Geometry check sheet. Reference: drawing and pictorial views, mm from the part's lowest x, y, z. Give positions to 0.01 mm unless a question says otherwise; leave off trailing zeros. Write each loop counter-clockwise with the first axis right and the second up, starting at its lowest first coordinate (ties: lowest second). Pieces come first, ordered by that corner, then holes. Notation, with made-up numbers: (81, 43.5) -> (96, 43.5) arc R20 cw to (96, 70.5) -> close; hole circle Ø2 at (31, 46.5). An arc over 180 degrees is marked (long way). Use a Markdown table: item, result. Add a question column.
1. Scan lines: probe 1 along Y at (x, z) = (24.5, 1.85); probe 2 along X at (y, z) = (3.25, 1.35). Record each from-to range of solid material in increasing order. Write a range as [from, to].
2. Gauge pin test, flat ends, axial feed: P1, Ø1, axis at x = 25.5, z = 3.5, coming from the -Y side; P2, Ø0.7, axis at y = 8, z = 3.5, coming from the +X side. Record the tip position at first contact, or that the pin passes through.
3. Cross-section at C-C (y = 3). Enter the section's corners in (x, z).
4. Release check for a two-part mould opening along Y. For the marked faces 1, 2, 3 and 4 record: released by +Y, released by -Y, zero draft, split by the parting line, or undercut.
5. Cross-section at A-A (x = 24.25). Enter the section's corners in (y, z), then the cut area to 3 significant figures.
6. Cross-section at B-B (z = 0.6). Enter the section's corners in (x, y).
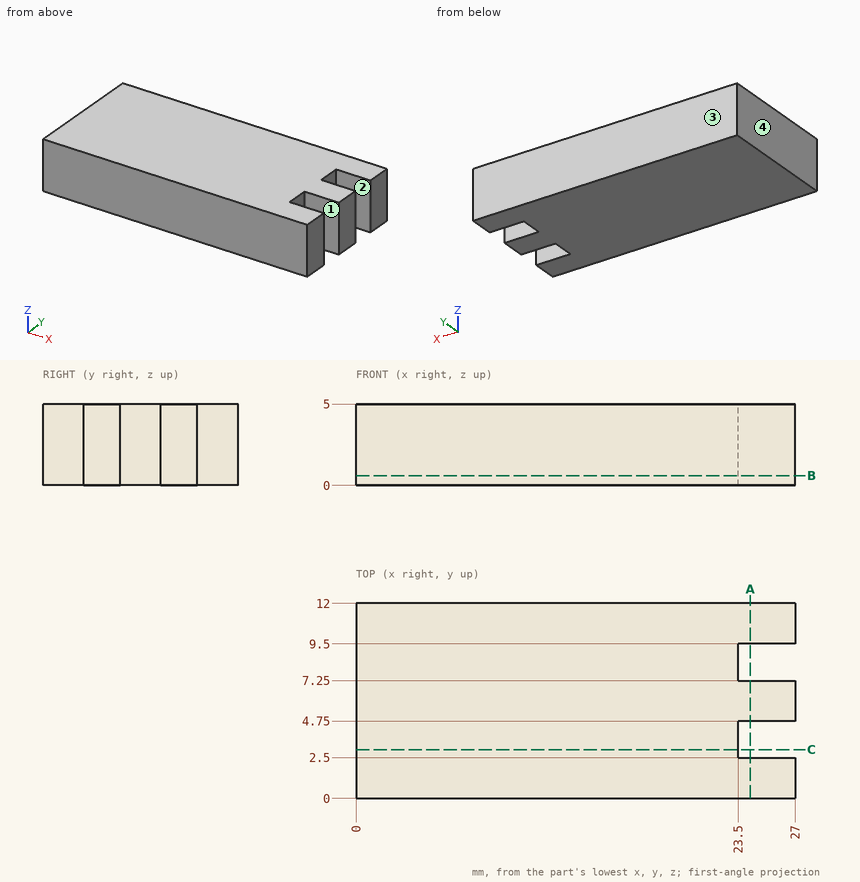
Worked answers:
| question | item | result |
|---|---|---|
| 1 | probe 1 | y = [0, 2.5], [4.75, 7.25], [9.5, 12] |
| 1 | probe 2 | x = [0, 23.5] |
| 2 | P1 | stops at y = 0 |
| 2 | P2 | stops at x = 23.5 |
| 3 | outline | (0, 0) -> (23.5, 0) -> (23.5, 5) -> (0, 5) -> close |
| 4 | face 1 | undercut |
| 4 | face 2 | undercut |
| 4 | face 3 | released by +Y |
| 4 | face 4 | zero draft |
| 5 | outline | (0, 0) -> (2.5, 0) -> (2.5, 5) -> (0, 5) -> close; (4.75, 0) -> (7.25, 0) -> (7.25, 5) -> (4.75, 5) -> close; (9.5, 0) -> (12, 0) -> (12, 5) -> (9.5, 5) -> close |
| 5 | area | 37.5 mm² |
| 6 | outline | (0, 0) -> (27, 0) -> (27, 2.5) -> (23.5, 2.5) -> (23.5, 4.75) -> (27, 4.75) -> (27, 7.25) -> (23.5, 7.25) -> (23.5, 9.5) -> (27, 9.5) -> (27, 12) -> (0, 12) -> close |
